Design review of the part shown in the three views and the two pictorial views. Dimensions are in mm from the part's minimum x, y and z. Round coordinates to 2 decimals unless told otherwise and drop trailing zeros. Write each loop counter-clockwise with the first axis right and the second up, starting at its lowest first coordinate (ties: lowest second). Pieces come first, ordered by that corner, then holes. Notation, with made-up numbers: (47.5, -27.75) - (100.5, -27.75) arc R23 cw to (100.5, -4.75) - close; hole circle Ø11 at (37.5, -6). An arc over 180 degrees is marked (long way). Use one line per item in the form item = value.
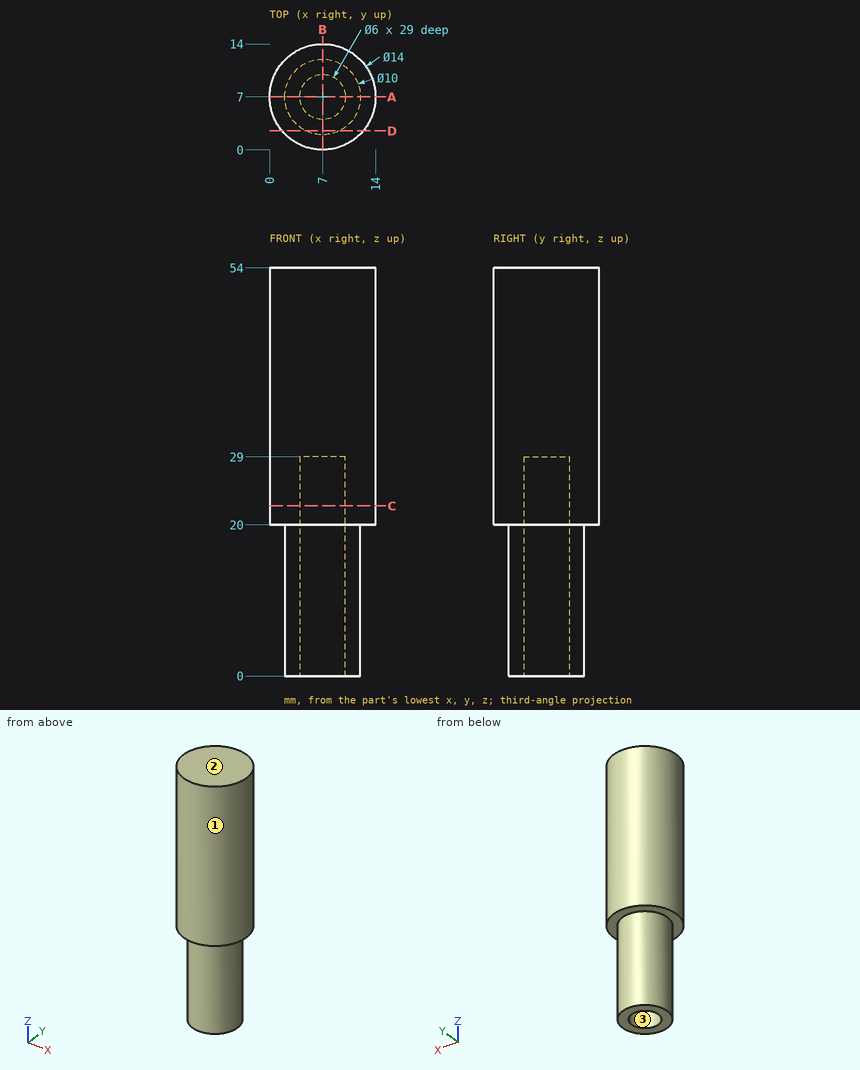
Q1. We need section D-D on y = 2.5. Write out the cut boundary in (x, z).
Calculated:
outline = (1.64, 20) - (4.82, 20) - (4.82, 0) - (9.18, 0) - (9.18, 20) - (12.36, 20) - (12.36, 54) - (1.64, 54) - close
Q2. We need section C-C on z = 22.5. Write out the cut boundary in (x, y).
Calculated:
outline = circle Ø14 at (7, 7); hole circle Ø6 at (7, 7)
Q3. To check wall thickness, follow line 1 along Y through (x, z) = (7, 8); line 2 along Z through (x, y) = (8.75, 6); line 3 along Z through (x, y) = (11.75, 4). State the ranges of each line that lie inside material, in increasing order. Write a range as from..to.
Calculated:
line_1 = 2..4, 10..12
line_2 = 29..54
line_3 = 20..54
Q4. For P1, Ø3, axis at x = 6, z = 12.5, coming from the +Y side; P2, Ø1, axis at y = 6.5, z = 7.5, coming from the +X side; P3, Ø1, axis at x = 11.5, z = 24, coming from the -Y side, all flat-tipped, find the tip position at first contact; note any pin that passes through.
Calculated:
P1 = 12
P2 = 12
P3 = 1.26
Q5. Draft analysis for pull direction X (two halves, no side actions). For the marked faces 1, 2 and 3, state which applies: released by +X, released by -X, zero draft, split by the parting line, or undercut.
Calculated:
face_1 = split by the parting line
face_2 = zero draft
face_3 = undercut
Q6. We need section A-A on y = 7. Write out the cut boundary in (x, z).
Calculated:
outline = (0, 20) - (2, 20) - (2, 0) - (4, 0) - (4, 29) - (10, 29) - (10, 0) - (12, 0) - (12, 20) - (14, 20) - (14, 54) - (0, 54) - close
